```python
from build123d import *
from build123d import SkipClean  # not in build123d's __all__

# Parameters (mm, degrees)
F1_DEPTH       = 10
F3_D           = 3.556
F3_CBORE_D     = 7.62
F3_CBORE_DEPTH = 10
F4_DEPTH       = 10.001
F6_D           = 3.556
F7_R           = 5


# Not quite as in the source:
# - a feature names something its author has since deleted; it is built from what else it names


with BuildPart() as f1:
    # F0 (on Top) → F1 (new body)
    with BuildSketch(Plane.XY):
        with BuildLine():
            ThreePointArc((16.1705551086, 23.468343518), (24.7491207645, 14.1326225939), (28.4297379517, 2))
            Line((28.4297379517, 2), (28.4297379517, 7))
            Line((28.4297379517, 7), (32.7604945018, 7))
            ThreePointArc((32.7604945018, 7), (26.8945535829, 19.9733068763), (16.1705551086, 29.3387652685))
            Line((16.1705551086, 29.3387652685), (16.1705551086, 23.468343518))
        make_face()
        with BuildLine():
            ThreePointArc((-16.1705551086, 23.468343518), (0, 28.5), (16.1705551086, 23.468343518))
            Line((16.1705551086, 23.468343518), (16.1705551086, 29.3387652685))
            Line((16.1705551086, 29.3387652685), (-16.1705551086, 29.3387652685))
            Line((-16.1705551086, 29.3387652685), (-16.1705551086, 23.468343518))
        make_face()
        with BuildLine():
            ThreePointArc((-28.4297379517, 2), (-24.7491207645, 14.1326225939), (-16.1705551086, 23.468343518))
            Line((-16.1705551086, 23.468343518), (-16.1705551086, 29.3387652685))
            ThreePointArc((-16.1705551086, 29.3387652685), (-26.8945535829, 19.9733068763), (-32.7604945018, 7))
            Line((-32.7604945018, 7), (-28.4297379517, 7))
            Line((-28.4297379517, 7), (-28.4297379517, 2))
        make_face()
        with BuildLine():
            Line((-48.4297379517, 2), (-33.4402452144, 2))
            ThreePointArc((-33.4402452144, 2), (-33.1946454228, 4.5128167765), (-32.7604945018, 7))
            Line((-32.7604945018, 7), (-48.4297379517, 7))
            Line((-48.4297379517, 7), (-48.4297379517, 2))
        make_face()
        with BuildLine():
            Line((-33.4402452144, 2), (-28.4297379517, 2))
            Line((-28.4297379517, 2), (-28.4297379517, 7))
            Line((-28.4297379517, 7), (-32.7604945018, 7))
            ThreePointArc((-32.7604945018, 7), (-33.1946454228, 4.5128167765), (-33.4402452144, 2))
        make_face()
        with BuildLine():
            Line((28.4297379517, 7), (28.4297379517, 2))
            Line((28.4297379517, 2), (33.4402452144, 2))
            ThreePointArc((33.4402452144, 2), (33.1946454228, 4.5128167765), (32.7604945018, 7))
            Line((32.7604945018, 7), (28.4297379517, 7))
        make_face()
        with BuildLine():
            ThreePointArc((32.7604945018, 7), (33.1946454228, 4.5128167765), (33.4402452144, 2))
            Line((33.4402452144, 2), (48.4297379517, 2))
            Line((48.4297379517, 2), (48.4297379517, 7))
            Line((48.4297379517, 7), (32.7604945018, 7))
        make_face()
        with BuildLine():
            Line((-16.1705551086, 33.5), (-16.1705551086, 29.3387652685))
            ThreePointArc((-16.1705551086, 29.3387652685), (-8.3486933282, 32.4430165014), (1.811e-07, 33.5))
            Line((1.811e-07, 33.5), (-16.1705551086, 33.5))
        make_face()
        with BuildLine():
            ThreePointArc((1.811e-07, 33.5), (8.3486935036, 32.4430164563), (16.1705551086, 29.3387652685))
            Line((16.1705551086, 29.3387652685), (16.1705551086, 33.5))
            Line((16.1705551086, 33.5), (1.811e-07, 33.5))
        make_face()
        with BuildLine():
            Line((-16.1705551086, 23.468343518), (16.1705551086, 23.468343518))
            ThreePointArc((16.1705551086, 23.468343518), (0, 28.5), (-16.1705551086, 23.468343518))
        make_face()
        Polygon((-16.1705551086, 33.5), (1.811e-07, 33.5), (16.1705551086, 33.5), (16.1705551086, 38.5), (-16.1705551086, 38.5), align=None)
        with BuildLine():
            Line((-16.1705551086, 29.3387652685), (16.1705551086, 29.3387652685))
            ThreePointArc((16.1705551086, 29.3387652685), (8.3486935036, 32.4430164563), (1.811e-07, 33.5))
            ThreePointArc((1.811e-07, 33.5), (-8.3486933282, 32.4430165014), (-16.1705551086, 29.3387652685))
        make_face()
    extrude(amount=F1_DEPTH)

    # F3 (through all)
    with Locations(Plane.XZ.offset(-23.468343518)):
        with Locations((0, 5)):
            CounterBoreHole(F3_D / 2, F3_CBORE_D / 2, F3_CBORE_DEPTH)

    # F0 (on Top) → F4 (cut, through all)
    with BuildSketch(Plane.XY):
        with BuildLine():
            Line((-16.1705551086, 23.468343518), (16.1705551086, 23.468343518))
            ThreePointArc((16.1705551086, 23.468343518), (0, 28.5), (-16.1705551086, 23.468343518))
        make_face()
    with SkipClean():  # cleaning this boolean's faces spoils the solid; the shape is the same uncleaned
        extrude(amount=F4_DEPTH, mode=Mode.SUBTRACT)

    # F6 (through all)
    with Locations(Plane.XZ.offset(-2)):
        with Locations((-39.116, 4.78035165), (39.116, 4.78035165)):
            Hole(F6_D / 2)

    # F7
    f7_edges = [f1.edges().sort_by_distance(p)[0] for p in [
        (-32.760495, 7, 5),
        (32.760495, 7, 5),
        (16.170555, 29.338765, 5),
        (-16.170555, 29.338765, 5),
    ]]
    fillet(f7_edges, radius=F7_R)


solid = f1.part
```
Can you work these out from the model? Positions are in its coordinate system, mm. A direction names the side the tool comes from. Coordinates: 2 decimals unless noted, no trailing zeros. Loops run counter-clockwise (first coordinate to the right, second up) from the corner with the lowest first, then second, coordinate; pieces in that order, holes last. Notation, with made-up numbers: (-1, -5) -> (21, -5) arc R29 cw to (21, 19) -> close; hole circle Ø3 at (80.25, -12.75). An arc over 180 degrees is marked (long way). Answer as a JSON object with one key per item and string values.
1) For P1, Ø4, axis at x = -24, y = 7, coming from the +Z side; P2, Ø5, axis at x = -40.5, z = 2.5, coming from the +Y side; P3, Ø4.5, axis at x = 0, z = 5, coming from the -Y side; P4, Ø1.9, axis at y = 34, z = 5, coming from the -X side, each with a flat end and sliding along its axis, tell me the tip position at first contact or that it passes through.
Results:
{"P1": "passes through", "P2": "stops at y = 7", "P3": "stops at y = 33.47", "P4": "stops at x = -16.17"}
2) Thinking about a two-plate mould opening in Z: for faces 1 (the face through (-4, 30, 10)), 2 (the face through (0.231, 36.019, 6.763)), 3 (the face through (1, 33.468, 3)), 4 (the face through (33.61, 7.98, 5.07)), which applies, pulls with the +Z half, pulls with the -Z half, needs draft (parallel to the pull), parting line crosses it, or undercut?
Results:
{"face 1": "pulls with the +Z half", "face 2": "undercut", "face 3": "undercut", "face 4": "needs draft"}
3) If I drill on line 1 (Z direction, x = 0, y = 30.7); line 2 (Y direction, x = 42.5, z = 2.25); line 3 (X direction, y = 4.5, z = 6), over which ranges is the centre line in solid material (lowest first)?
Results:
{"line 1": "z = 0 to 1.19, 8.81 to 10", "line 2": "y = 2 to 7", "line 3": "x = -48.43 to -40.41, -37.82 to -28.14, 28.14 to 37.82, 40.41 to 48.43"}
4) Imagine slicing it at A-A (x = 0). Please give me the cut outline in (y, z), then the cut area to 3 significant figures.
Results:
{"outline": "(28.5, 0) -> (38.5, 0) -> (38.5, 3.22) -> (33.47, 3.22) -> (33.47, 1.19) -> (28.5, 1.19) -> close; (28.5, 8.81) -> (33.47, 8.81) -> (33.47, 6.78) -> (38.5, 6.78) -> (38.5, 10) -> (28.5, 10) -> close", "area": "44.2 mm^2"}
5) For faces 5 (the face through (37.474, 4.535, 4.099)), 6 (the face through (1.76, 30.81, 1.62)), 7 (the face through (43, 7, 5)), 8 (the face through (-16.171, 35, 5)), which set-ups out of +Z, -Z, +X, -X, +Y, -Y let a thin tool reach every point of the face, with its end or its side?
Results:
{"face 5": "+Y, -Y", "face 6": "-Y", "face 7": "+Z, -Z, +X, +Y", "face 8": "+Z, -Z, -X, +Y"}
6) Imagine slicing it at B-B (y = 20.5). Please give me the cut outline in (x, z).
Results:
{"outline": "(-26.5, 0) -> (-19.8, 0) -> (-19.8, 10) -> (-26.5, 10) -> close; (19.8, 0) -> (26.5, 0) -> (26.5, 10) -> (19.8, 10) -> close"}
